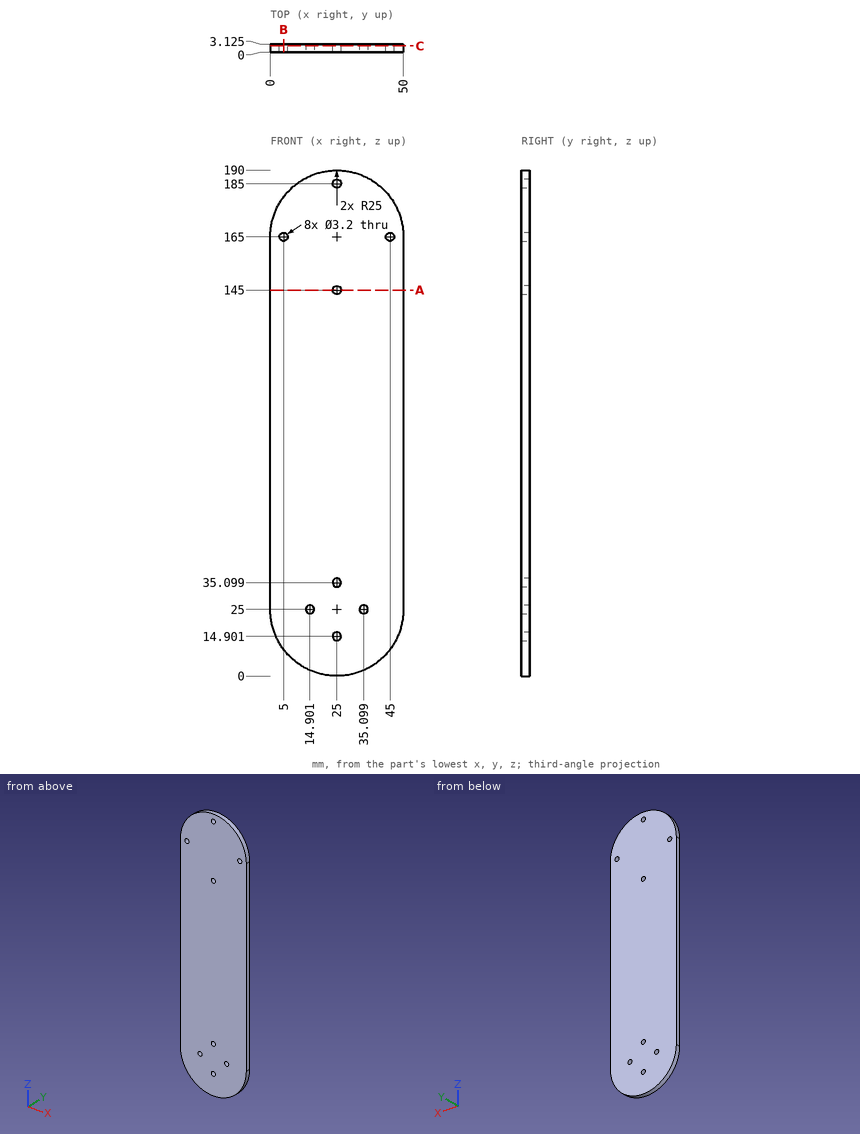
Print and shaded views of the part. All mm, measured from the part's lowest x, y and z. Round coordinates to 2 decimals unless told otherwise and drop trailing zeros. Write each loop counter-clockwise with the first axis right and the second up, starting at its lowest first coordinate (ties: lowest second). Pieces come first, ordered by that corner, then holes. Notation, with made-up numbers: (42, 8) - (73, 8) arc R13 cw to (73, 26) - close; hole circle Ø6 at (53, 33.5). An arc over 180 degrees is marked (long way). Use CSV: the item, a comma, the result in double quotes. Start each with the question number.
Item 1: Pin check, flat tip, straight feed: P1, Ø1.5, axis at x = 21, y = 1.5, coming from the +Z side. Stop position of the tip, or through.
Item 2: Band-saw the part on C-C (y = 2.45). State how many separate pieces and enclosed holes the cut face has, and give its area (3 significant figures).
Item 3: Drill centre lines: L1, parallel to X at y = 1.35, z = 25; L2, parallel to X at y = 2.45, z = 26; L3, parallel to Z at x = 36.5, y = 2.85 (1 decimal). Where is each one in solid material? Low to high. Write a range as [from, to].
Item 4: Band-saw the part on B-B (x = 5). Write the cut outline in (y, z) (1 decimal).
Item 5: Band-saw the part on A-A (z = 145). Write the cut outline in (x, y) (1 decimal), and give its area (3 significant figures).
Checked values:
1,P1,"stops at z = 189.79"
2,separate pieces,"1"
2,enclosed holes,"8"
2,area,"8,900 mm²"
3,L1,"x = [0, 13.3], [16.5, 33.5], [36.7, 50]"
3,L2,"x = [0, 13.65], [16.15, 33.85], [36.35, 50]"
3,L3,"z = [2.8, 24.2], [25.8, 187.2]"
4,outline,"(0, 10) - (3.1, 10) - (3.1, 163.4) - (0, 163.4) - close; (0, 166.6) - (3.1, 166.6) - (3.1, 180) - (0, 180) - close"
5,outline,"(0, 0) - (23.4, 0) - (23.4, 3.1) - (0, 3.1) - close; (26.6, 0) - (50, 0) - (50, 3.1) - (26.6, 3.1) - close"
5,area,"146 mm²"
